Work out the finished part from the listing and answer in its coordinate system (mm). Face numbers are marked on the shaded views. A direction names the side the tool comes from. Round coordinates to 2 decimals unless told otherwise and drop trailing zeros. Write each loop counter-clockwise with the first axis right and the second up, starting at its lowest first coordinate (ties: lowest second). Pieces come first, ordered by that corner, then holes.
1. Find section D-D (y = 1.5). Write down the section's boundary in (x, z), and give its area (3 significant figures).
2. Find section C-C (z = 5). Write down the section's boundary in (x, y), and give its area (3 significant figures).
3. Find section B-B (x = 1). Write down the section's boundary in (y, z), and give its area (3 significant figures).
4. Flat-ended cylindrical pins translate along their axes: pin 1 Ø6.5 at (x, z) = (-5, 1.5) entering from +Y; pin 2 Ø1 at (y, z) = (2, -7.5) entering from -X; pin 3 Ø3 at (x, y) = (-5.5, 3.5) entering from +Z. Find the tip coordinate at first contact, or state that the pin passes through.
5. Find section A-A (z = -2.5). Write down the section's boundary in (x, y), and give its area (3 significant figures).
6. Straight lines are drawn through the part: probe 1 along Z at (x, y) = (-7.35, 0.45); probe 2 along X at (y, z) = (0.65, 2); probe 3 along X at (y, z) = (0.6, -8). For each, find the intervals that lie inside material, in ascending order.
7. A tool of negligible diameter and unlimited length cuts with its end or side. For the marked faces 1, 2 and 3, from which of +Z, -Z, +X, -X, +Y, -Y can it reach the whole face along a straight path? Write none if from no direction.
Autodesk Inventor part; units mm, degrees
ref_plane "YZ Plane" through (0, 0, 0) normal (1, 0, 0) x (0, 1, 0)
ref_plane "XZ Plane" through (0, 0, 0) normal (0, 1, 0) x (-1, 0, 0)
ref_plane "XY Plane" through (0, 0, 0) normal (0, 0, 1) x (1, 0, 0)
sketch "Sketch1" plane through (0, 0, 0) normal (0, 1, 0) x (-1, 0, 0)
  line L0 (-12.35, 10.5) -> (12.35, 10.5)
  line L1 (12.35, 10.5) -> (12.35, -10.5)
  line L2 (12.35, -10.5) -> (-12.35, -10.5)
  line L3 (-12.35, -10.5) -> (-12.35, 10.5)
  line L4 (-12.35, 10.5) -> (12.35, -10.5) construction
  line L5 (12.35, 10.5) -> (-12.35, -10.5) construction
  point P0 (0, 0)
  dimension "d0" = 21
  dimension "d1" = 24.7
extrude "Extrusion1" add sketch "Sketch1" along normal blind 1
sketch "Sketch2" plane through (0, 1, 0) normal (0, 1, 0) x (1, 0, 0)
  circle A0 centre (-10.35, 2.5) radius 1
  line L0 (12.35, 10.5) -> (-12.35, 10.5)
  line L1 (-12.35, 10.5) -> (-12.35, -10.5)
  point P0 (0, 0)
  dimension "d4" = 2
  dimension "d5" = 8
  dimension "d6" = 2
extrude "Extrusion2" cut sketch "Sketch2" against normal blind 1
sketch "Sketch3" plane through (0, 1, 0) normal (0, 1, 0) x (1, 0, 0)
  circle A0 centre (-4.35, 6.5) radius 3
  line L0 (-12.35, 10.5) -> (-12.35, -10.5)
  line L1 (12.35, 10.5) -> (-12.35, 10.5)
  line L2 (0, 0) -> (0, 10.5) construction
  circle A1 centre (4.35, 6.5) radius 3
  dimension "d9" = 6
  dimension "d10" = 8
  dimension "d11" = 4
extrude "Extrusion3" add sketch "Sketch3" along normal blind 6
fillet "Fillet1" radius 0.2 2 edges at (-7.35, 7, -6.5) (1.35, 7, -6.5)
sketch "Sketch4" plane through (0, 1, 0) normal (0, 1, 0) x (1, 0, 0)
  circle A0 centre (-7.35, 1) radius 0.5
  circle A1 centre (-7.35, -2) radius 0.5
  circle A2 centre (-10.35, 2.5) radius 1
  line L0 (-10.35, 1.5) -> (-7.35, 1.5) construction
  circle A3 centre (-7.35, -5) radius 0.5
  circle A4 centre (-7.35, -8) radius 0.5
  circle A5 centre (-4.35, 6.5) radius 3
  line L1 (-7.35, 6.5) -> (-7.35, 1.5) construction
  line L2 (0, 0) -> (0, -10.5851) construction
  circle A6 centre (7.35, 1) radius 0.5
  circle A7 centre (7.35, -2) radius 0.5
  circle A8 centre (7.35, -5) radius 0.5
  circle A9 centre (7.35, -8) radius 0.5
  dimension "d15" = 1
  dimension "d16" = 1
  dimension "d17" = 1
  dimension "d18" = 1
  dimension "d19" = 3
  dimension "d20" = 3
  dimension "d21" = 3
extrude "Extrusion4" cut sketch "Sketch4" against normal blind 1 contours A0 | A1 | A3 | A4 | A6 | A7 | A8 | A9
sketch "Sketch5" plane through (0, 1, 0) normal (0, 1, 0) x (1, 0, 0)
  line L0 (-2, 1) -> (2, 1)
  line L1 (2, 1) -> (2, -8)
  line L2 (2, -8) -> (-2, -8)
  line L3 (-2, -8) -> (-2, 1)
  circle A0 centre (-7.35, 1) radius 0.5
  point P0 (0, 0)
  point P1 (0, 1)
  dimension "d26" = 4
  dimension "d27" = 9
extrude "Extrusion5" add sketch "Sketch5" along normal blind 1 contours L0 L1 L2 L3
chamfer "Chamfer1" distance 0.2 angle 45 2 edges at (2, 2, 3.5) (-2, 2, 3.5)
sketch "Sketch6" plane through (0, 1, 0) normal (0, 1, 0) x (1, 0, 0)
  circle A0 centre (-10.85, 8) radius 0.5
  circle A1 centre (-10.85, 5) radius 0.5
  line L0 (12.35, 10.5) -> (-12.35, 10.5)
  line L1 (-12.35, 10.5) -> (-12.35, -10.5)
  point P0 (0, 0)
  dimension "d33" = 1
  dimension "d34" = 1
  dimension "d35" = 2.5
  dimension "d36" = 1.5
  dimension "d37" = 3
extrude "Extrusion6" cut sketch "Sketch6" against normal blind 1
sketch "Sketch7" plane through (0, 1, 0) normal (0, 1, 0) x (1, 0, 0)
  line L0 (-9.7434, 8.3067) -> (-6.693, 8.3067) construction
  line L1 (-6.693, 8.3067) -> (-6.693, 5.9132) construction
  line L2 (-6.693, 5.9132) -> (-9.7434, 5.9132) construction
  line L3 (-9.7434, 5.9132) -> (-9.7434, 8.3067) construction
  line L4 (-9.6683, 5.4228) -> (-8.67, 5.4228) construction
  line L5 (-8.67, 5.4228) -> (-8.67, 5.1797) construction
  line L6 (-8.67, 5.1797) -> (-9.6683, 5.1797) construction
  line L7 (-9.6683, 5.1797) -> (-9.6683, 5.4228) construction
  line L8 (-8.848, 7.8602) -> (-9.1867, 7.8602)
  line L9 (-9.1867, 7.8602) -> (-9.1867, 7.5214)
  line L10 (-9.1867, 7.5214) -> (-9.2985, 7.5214)
  line L11 (-9.2985, 7.5214) -> (-9.2985, 7.8602)
  line L12 (-9.2985, 7.8602) -> (-9.6373, 7.8602)
  line L13 (-9.6373, 7.8602) -> (-9.6373, 7.9679)
  line L14 (-9.6373, 7.9679) -> (-9.2985, 7.9679)
  line L15 (-9.2985, 7.9679) -> (-9.2985, 8.3067)
  line L16 (-9.2985, 8.3067) -> (-9.1867, 8.3067)
  line L17 (-9.1867, 8.3067) -> (-9.1867, 7.9679)
  line L18 (-9.1867, 7.9679) -> (-8.848, 7.9679)
  line L19 (-8.848, 7.9679) -> (-8.848, 7.8602)
  line L20 (-8.7899, 5.1797) -> (-9.5468, 5.1797)
  line L21 (-9.5468, 5.1797) -> (-9.5468, 5.4228)
  line L22 (-9.5468, 5.4228) -> (-8.7899, 5.4228)
  line L23 (-8.7899, 5.4228) -> (-8.7899, 5.1797)
  point P0 (0, 0)
emboss "Emboss1" sketch "Sketch7" operation add depth 0.1 direction (0, -1, 0)
properties part number "L298N_CPY"
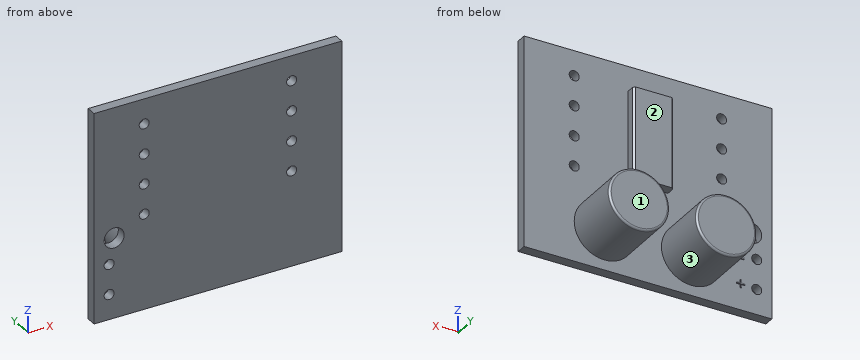
Worked answers:
1. outline: circle Ø6 at (-4.35, -6.5); (-2, -1) - (2, -1) - (2, 8) - (-2, 8) - close; circle Ø6 at (4.35, -6.5)
1. area: 92.5 mm2
2. outline: (-12.35, 0) - (-7.85, 0) - (-7.85, 1) - (-12.35, 1) - close; (-6.85, 0) - (6.85, 0) - (6.85, 1) - (2, 1) - (2, 1.8) - (1.8, 2) - (-1.8, 2) - (-2, 1.8) - (-2, 1) - (-6.85, 1) - close; (7.85, 0) - (12.35, 0) - (12.35, 1) - (7.85, 1) - close
2. area: 26.7 mm2
3. outline: (0, -10.5) - (1, -10.5) - (1, -1) - (2, -1) - (2, 8) - (1, 8) - (1, 10.5) - (0, 10.5) - close
3. area: 30.0 mm2
4. pin 1: stops at y = 2
4. pin 2: stops at x = -7.31
4. pin 3: stops at z = -3.5
5. outline: (-12.35, 0) - (-11.35, 0) - (-11.35, 1) - (-12.35, 1) - close; (-9.35, 0) - (12.35, 0) - (12.35, 1) - (-9.35, 1) - close
5. area: 22.7 mm2
6. probe 1: z = -10.5 to -1.5, -0.5 to 1.5, 2.5 to 4.5, 5.5 to 7.5, 8.5 to 10.5
6. probe 2: x = -12.35 to -7.85, -6.85 to 6.85, 7.85 to 12.35
6. probe 3: x = -12.35 to -11.35, -10.35 to 12.35
7. face 1: +Z, -Z, +X, -X, +Y
7. face 2: +Z, +X, -X, +Y
7. face 3: +Y
